Work out the finished part from the listing and answer in its coordinate system (mm). Face numbers are marked on the shaded views. A direction names the side the tool comes from. Coordinates: 2 decimals unless noted, no trailing zeros. Order: outer loops, then holes, each group sorted by start corner. A loop starts at its lowest first (then second) coordinate and runs counter-clockwise, first axis right, second up. Notation, with made-up numbers: M 34,-16.75 L 60,-16.75 A11 ccw 60,-11.75 Z; hole C 1.5,74 d5. An arc over 180 degrees is marked long. Use a Markdown table: item, result.
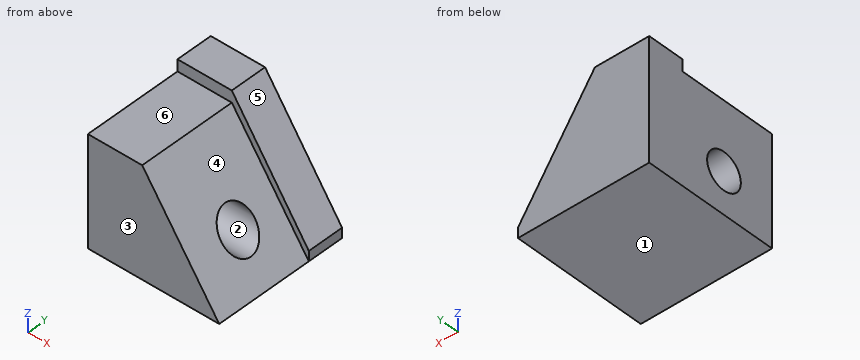
from build123d import *

# Parameters (mm, degrees)
F0_W     = 135.070444
F0_H     = 139.326424
F1_DEPTH = 124.714
F3_DEPTH = 101.6
F5_DEPTH = 101.6
F7_DEPTH = 50.8
F8_R     = 19.086434
F9_DEPTH = 138.176


with BuildPart() as f1:
    # F0 (on Top) → F1 (new body)
    with BuildSketch(Plane.XY):
        Rectangle(F0_W, F0_H)
    extrude(amount=F1_DEPTH)

    # F2 (on face) → F3 (cut, symmetric)
    with BuildSketch(Plane.XZ.offset(69.663212)):
        Polygon((67.535222, 124.714), (-20.09901, 124.714), (67.535222, 0), align=None)
    extrude(amount=F3_DEPTH, both=True, mode=Mode.SUBTRACT)

    # F4 (on face) → F5 (cut)
    with BuildSketch(Plane.XZ.offset(69.663212)):
        Polygon((-67.535222, 112.750193), (-11.692263, 112.750193), (-20.09901, 124.714), (-67.535222, 124.714), align=None)
    extrude(amount=-F5_DEPTH, mode=Mode.SUBTRACT)

    # F6 (on face) → F7 (cut)
    with BuildSketch(Plane.XZ.offset(-31.936788)):
        Polygon((67.535222, 124.714), (-11.692263, 124.714), (67.535222, 10.252971), align=None)
    extrude(amount=-F7_DEPTH, mode=Mode.SUBTRACT)

    # F8 (on Right) → F9 (cut, symmetric)
    with BuildSketch(Plane.YZ):
        with Locations((-15.093137, 43.024112)):
            Circle(F8_R)
    extrude(amount=F9_DEPTH, both=True, mode=Mode.SUBTRACT)


solid = f1.part
1. For the marked faces 4, 5 and 6, determine the directions among +Z, -Z, +X, -X, +Y, -Y from which every point of the face is accessible in a straight line to the end or side of a thin tool.
Answers below:
| item | result |
|---|---|
| face 4 | +Z, +X, -Y |
| face 5 | +Z, +X, +Y, -Y |
| face 6 | +Z, +X, -X, -Y |
2. Flat-ended cylindrical pins translate along their axes: P1, Ø3, axis at x = 19, y = 13, coming from the +Z side; P2, Ø5, axis at y = 15.5, z = 52.5, coming from the +X side. Find the tip coordinate at first contact, or state that the pin passes through.
Answers below:
| item | result |
|---|---|
| P1 | z = 71.21 |
| P2 | x = 32.4 |
3. Section B-B on y = -17.5 is taken. Determine the outline of the cut face in (x, z), then the cut area to 3 significant figures.
Answers below:
| item | result |
|---|---|
| outline | M -67.54,0 L 67.54,0 L 50.61,24.09 L -67.54,24.09 Z; M -67.54,61.96 L 24,61.96 L -11.69,112.75 L -67.54,112.75 Z |
| area | 6,790 mm² |
4. Section C-C on x = 10.5 is taken. Determine the outline of the cut face in (y, z), then the cut area to 3 significant figures.
Answers below:
| item | result |
|---|---|
| outline | M -69.66,0 L 69.66,0 L 69.66,92.65 L 31.94,92.65 L 31.94,81.17 L -69.66,81.17 Z; hole C -15.09,43.02 d38.17 |
| area | 10,600 mm² |
5. For a pull along Y with two mould halves and no side action, classify the marked faces 1, 2 and 3 as +Y half, -Y half, draft (parallel to the pull), parting line (faces both ways), or undercut.
Answers below:
| item | result |
|---|---|
| face 1 | draft |
| face 2 | undercut |
| face 3 | -Y half |
6. Section D-D on x = 27 is taken. Determine the outline of the cut face in (y, z).
Answers below:
| item | result |
|---|---|
| outline | M -69.66,0 L 69.66,0 L 69.66,68.81 L 31.94,68.81 L 31.94,57.69 L -2.87,57.69 A19.09 cw long -27.31,57.69 L -69.66,57.69 Z |
7. Section A-A on z = 47 is taken. Determine the outline of the cut face in (x, y).
Answers below:
| item | result |
|---|---|
| outline | M -67.54,-69.66 L 34.51,-69.66 L 34.51,-33.76 L -67.54,-33.76 Z; M -67.54,3.57 L 34.51,3.57 L 34.51,31.94 L 42.1,31.94 L 42.1,69.66 L -67.54,69.66 Z |
8. Find the intervals of material crossed by probe 1 along Z at (x, y) = (-55.5, -15); probe 2 along Z at (x, y) = (-22.5, 9.5); probe 3 along Y at (x, z) = (-3.5, 105.5), in increasing order.
Answers below:
| item | result |
|---|---|
| probe 1 | 0 to 23.94, 62.11 to 112.75 |
| probe 2 | 0 to 112.75 |
| probe 3 | 31.94 to 69.66 |
